Source: three-view drawing plus pictorial views. Frame: mm from the lowest corner of the part. A direction names the side the tool comes from. Round coordinates to 2 decimals unless told otherwise and drop trailing zeros. Loops run counter-clockwise (first coordinate to the right, second up) from the corner with the lowest first, then second, coordinate; pieces in that order, holes last. Notation, with made-up numbers: (10, -8.5) -> (31, -8.5) arc R35 cw to (31, 29.5) -> close; hole circle Ø8 at (20, 62.5). An arc over 180 degrees is marked (long way). One line per question, with ' | ' between items. Start each with the question number.
Q1. Contact query for flat-ended pins moving along their axis: P1, Ø4, axis at x = 45.5, z = 7.5, coming from the -Y side; P2, Ø12, axis at x = 52.5, z = 25.5, coming from the +Y side; P3, Ø1.5, axis at x = 51.5, y = 13, coming from the -Z side. Output: stop coordinate, or through.
Q2. Cut plane A-A on y = 22.5. Return loops of the section in (x, z), and give its area (3 significant figures).
Q3. Material intervals for L1, parallel to X at y = 18.5, z = 38.5; L2, parallel to X at y = 27, z = 31; L3, parallel to X at y = 41.5, z = 34, sorted ascending.
Q4. Cut plane C-C on y = 41. Return loops of the section in (x, z), and give its area (3 significant figures).
Q5. Mould query, pull axis Y, two halves, no side actions, for the marked faces 1, 2 and 3. Classes: pulls with the +Y half, pulls with the -Y half, needs draft (parallel to the pull), parting line crosses it, or undercut.
Q6. Cut plane D-D on x = 69. Return loops of the section in (y, z).
Q7. Access query for the marked faces 4, 5 and 6. Directions: +Z, -Z, +X, -X, +Y, -Y. A direction counts if a zero-diameter tool reaches every point of the face in a straight line with its end or side. Return the directions, or none.
Q8. Cut plane B-B on z = 22.5. Return loops of the section in (x, y), and give its area (3 significant figures).
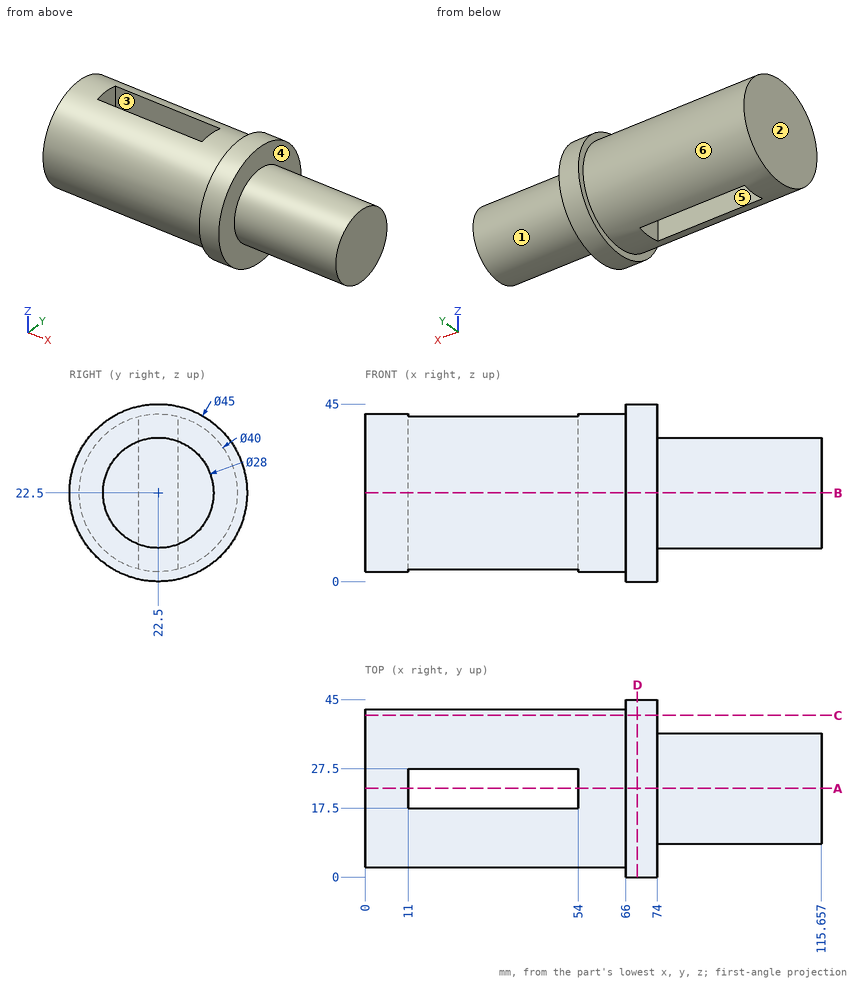
Results:
1) P1: y = 7.3 | P2: y = 42.5 | P3: z = 4.52
2) outline: (0, 2.5) -> (11, 2.5) -> (11, 42.5) -> (0, 42.5) -> close; (54, 2.5) -> (66, 2.5) -> (66, 0) -> (74, 0) -> (74, 8.5) -> (115.66, 8.5) -> (115.66, 36.5) -> (74, 36.5) -> (74, 45) -> (66, 45) -> (66, 42.5) -> (54, 42.5) -> close | area: 2,450 mm^2
3) L1: 0 to 11, 54 to 74 | L2: 0 to 11, 54 to 115.66 | L3: 66 to 74
4) outline: (0, 14.9) -> (66, 14.9) -> (66, 9.69) -> (74, 9.69) -> (74, 35.31) -> (66, 35.31) -> (66, 30.1) -> (0, 30.1) -> close | area: 1,210 mm^2
5) face 1: parting line crosses it | face 2: needs draft | face 3: undercut
6) outline: circle Ø45 at (22.5, 22.5)
7) face 4: +X | face 5: +Z, -Z | face 6: -X
8) outline: (0, 2.5) -> (66, 2.5) -> (66, 0) -> (74, 0) -> (74, 8.5) -> (115.66, 8.5) -> (115.66, 36.5) -> (74, 36.5) -> (74, 45) -> (66, 45) -> (66, 42.5) -> (0, 42.5) -> close; hole (11, 17.5) -> (54, 17.5) -> (54, 27.5) -> (11, 27.5) -> close | area: 3,740 mm^2
